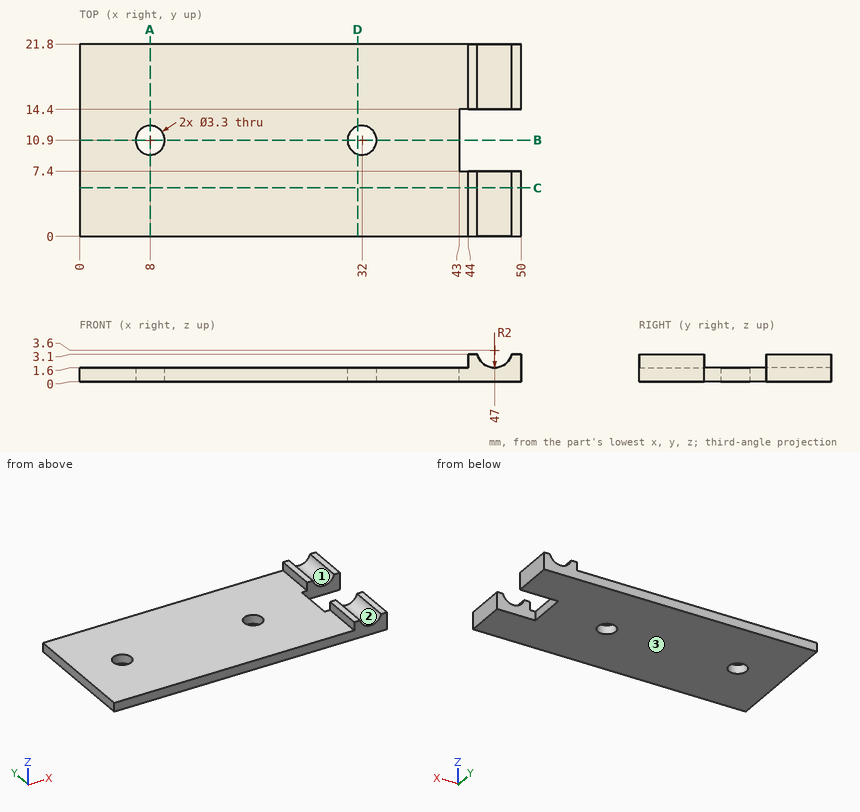
Geometry check sheet. Reference: drawing and pictorial views, mm from the part's lowest x, y, z. Round coordinates to 2 decimals unless told otherwise and drop trailing zeros. Loops run counter-clockwise (first coordinate to the right, second up) from the corner with the lowest first, then second, coordinate; pieces in that order, holes last. Notation, with made-up numbers: (20, 3.25) -> (72, 3.25) arc R20 ccw to (72, 29.25) -> close; hole circle Ø11 at (-4, 32). An arc over 180 degrees is marked (long way). Answer as a JSON object with one key per item and string values.
Q1. Scan lines: line 1 (Y direction, x = 8, z = 0.75); line 2 (X direction, y = 10.5, z = 1.55); line 3 (X direction, y = 9.75, z = 1.35). Record each from-to range of solid material in increasing order. Write a range as from..to.
Data:
{"line 1": "y = 0..9.25, 12.55..21.8", "line 2": "x = 0..6.4, 9.6..30.4, 33.6..43", "line 3": "x = 0..6.82, 9.18..30.82, 33.18..43"}
Q2. Go/stop test with flat-tipped pins: P1, Ø6, axis at x = 11, y = 6.5, coming from the +Z side; P2, Ø1.3, axis at y = 11.5, z = 0.5, coming from the +X side; P3, Ø1.6, axis at y = 3, z = 2.5, coming from the -X side. Record where each tip stops, or that it passes through.
Data:
{"P1": "stops at z = 1.6", "P2": "stops at x = 43", "P3": "stops at x = 44"}
Q3. Section check A-A (x = 8). Record the boundary of the cut face in (y, z).
Data:
{"outline": "(0, 0) -> (9.25, 0) -> (9.25, 1.6) -> (0, 1.6) -> close; (12.55, 0) -> (21.8, 0) -> (21.8, 1.6) -> (12.55, 1.6) -> close"}
Q4. Section check C-C (y = 5.5). Record the boundary of the cut face in (x, z), then the cut area to 3 significant figures.
Data:
{"outline": "(0, 0) -> (50, 0) -> (50, 3.1) -> (48.94, 3.1) arc R2 cw to (45.06, 3.1) -> (44, 3.1) -> (44, 1.6) -> (0, 1.6) -> close", "area": "84.7 mm2"}
Q5. Section check D-D (x = 31.5). Record the boundary of the cut face in (y, z), then the cut area to 3 significant figures.
Data:
{"outline": "(0, 0) -> (9.33, 0) -> (9.33, 1.6) -> (0, 1.6) -> close; (12.47, 0) -> (21.8, 0) -> (21.8, 1.6) -> (12.47, 1.6) -> close", "area": "29.8 mm2"}
Q6. Section check B-B (y = 10.9). Record the boundary of the cut face in (x, z), then the cut area to 3 significant figures.
Data:
{"outline": "(0, 0) -> (6.35, 0) -> (6.35, 1.6) -> (0, 1.6) -> close; (9.65, 0) -> (30.35, 0) -> (30.35, 1.6) -> (9.65, 1.6) -> close; (33.65, 0) -> (43, 0) -> (43, 1.6) -> (33.65, 1.6) -> close", "area": "58.2 mm2"}
Q7. Draft check along X on the marked faces 1, 2 and 3. Enter one of: pulls with the +X half, pulls with the -X half, needs draft (parallel to the pull), parting line crosses it, or undercut.
Data:
{"face 1": "undercut", "face 2": "undercut", "face 3": "needs draft"}
